Geometry check sheet. Reference: the model listing, model coordinates, mm. Give positions to 0.01 mm unless a question says otherwise; leave off trailing zeros. One line per item, written item: value. Start each with the question number.
(1) Sectioned sample at A-A, the plane z = 2.55. State how many separate pieces and enclosed holes the cut face has, then the cut area to 3 significant figures.
(2) Gauge pin test, flat ends, axial feed: pin 1 Ø1 at (y, z) = (102, 2.5) entering from +X; pin 2 Ø1.6 at (x, z) = (62, 1) entering from -Y; pin 3 Ø1 at (x, z) = (-61.5, 1) entering from +Y. Record the tip position at first contact, or that the pin passes through.
(3) Scan lines: line 1 along Y through (x, z) = (-54.5, 1.15); line 2 along X through (y, z) = (-150, 1.2). Record each from-to range of solid material in increasing order. Write a range as from..to.
from build123d import *

# Parameters (mm, degrees)
CROQUIS1_W              = 3.3
CROQUIS1_H              = 3.3
SALIENTE_EXTRUIR1_DEPTH = 3.3


with BuildPart() as part:
    # Croquis1 → Saliente-Extruir1 (new body)
    with BuildSketch(Plane.XY):
        Polygon((60, 27.9389154), (63.3, 27.9389154), (63.3, 19.9089154), (60, 19.9089154), (60, 11.03980694), (63.3, 11.03980694), (63.3, 3.00980694), (60, 3.00980694), (60, -3.00980694), (63.3, -3.00980694), (63.3, -11.03980694), (60, -11.03980694), (60, -19.9089154), (63.3, -19.9089154), (63.3, -27.9389154), (60, -27.9389154), (60, -36.80802386), (63.3, -36.80802386), (63.3, -44.83802386), (60, -44.83802386), (60, -53.70713232), (63.3, -53.70713232), (63.3, -61.73713232), (60, -61.73713232), (60, -70.60624078), (63.3, -70.60624078), (63.3, -78.63624078), (60, -78.63624078), (60, -87.50534924), (63.3, -87.50534924), (63.3, -95.53534924), (60, -95.53534924), (60, -104.4044577), (63.3, -104.4044577), (63.3, -112.4344577), (60, -112.4344577), (60, -121.30356616), (63.3, -121.30356616), (63.3, -129.33356616), (60, -129.33356616), (60, -138.20267462), (63.3, -138.20267462), (63.3, -146.23267462), (60, -146.23267462), (60, -155.10178308), (63.3, -155.10178308), (63.3, -163.13178308), (60, -163.13178308), (60, -172.00089154), (63.3, -172.00089154), (63.3, -180.03089154), (60, -180.03089154), (60, -188.9), (63.3, -188.9), (63.3, -196.93), (60, -196.93), (60, -200), (-60, -200), (-60, -196.93), (-63.3, -196.93), (-63.3, -188.9), (-60, -188.9), (-60, -180.03089154), (-63.3, -180.03089154), (-63.3, -172.00089154), (-60, -172.00089154), (-60, -163.13178308), (-63.3, -163.13178308), (-63.3, -155.10178308), (-60, -155.10178308), (-60, -146.23267462), (-63.3, -146.23267462), (-63.3, -138.20267462), (-60, -138.20267462), (-60, -129.33356616), (-63.3, -129.33356616), (-63.3, -121.30356616), (-60, -121.30356616), (-60, -112.4344577), (-63.3, -112.4344577), (-63.3, -104.4044577), (-60, -104.4044577), (-60, -95.53534924), (-63.3, -95.53534924), (-63.3, -87.50534924), (-60, -87.50534924), (-60, -78.63624078), (-63.3, -78.63624078), (-63.3, -70.60624078), (-60, -70.60624078), (-60, -61.73713232), (-63.3, -61.73713232), (-63.3, -53.70713232), (-60, -53.70713232), (-60, -44.83802386), (-63.3, -44.83802386), (-63.3, -36.80802386), (-60, -36.80802386), (-60, -27.9389154), (-63.3, -27.9389154), (-63.3, -19.9089154), (-60, -19.9089154), (-60, -11.03980694), (-63.3, -11.03980694), (-63.3, -3.00980694), (-60, -3.00980694), (-60, 3.00980694), (-63.3, 3.00980694), (-63.3, 11.03980694), (-60, 11.03980694), (-60, 19.9089154), (-63.3, 19.9089154), (-63.3, 27.9389154), (-60, 27.9389154), (-60, 36.80802386), (-63.3, 36.80802386), (-63.3, 44.83802386), (-60, 44.83802386), (-60, 53.70713232), (-63.3, 53.70713232), (-63.3, 61.73713232), (-60, 61.73713232), (-60, 70.60624078), (-63.3, 70.60624078), (-63.3, 78.63624078), (-60, 78.63624078), (-60, 87.50534924), (-63.3, 87.50534924), (-63.3, 95.53534924), (-60, 95.53534924), (-60, 104.4044577), (-63.3, 104.4044577), (-63.3, 112.4344577), (-60, 112.4344577), (-60, 121.30356616), (-63.3, 121.30356616), (-63.3, 129.33356616), (-60, 129.33356616), (-60, 138.20267462), (-63.3, 138.20267462), (-63.3, 146.23267462), (-60, 146.23267462), (-60, 155.10178308), (-63.3, 155.10178308), (-63.3, 163.13178308), (-60, 163.13178308), (-60, 172.00089154), (-63.3, 172.00089154), (-63.3, 180.03089154), (-60, 180.03089154), (-60, 188.9), (-63.3, 188.9), (-63.3, 196.93), (-60, 196.93), (-60, 200), (60, 200), (60, 196.93), (63.3, 196.93), (63.3, 188.9), (60, 188.9), (60, 180.03089154), (63.3, 180.03089154), (63.3, 172.00089154), (60, 172.00089154), (60, 163.13178308), (63.3, 163.13178308), (63.3, 155.10178308), (60, 155.10178308), (60, 146.23267462), (63.3, 146.23267462), (63.3, 138.20267462), (60, 138.20267462), (60, 129.33356616), (63.3, 129.33356616), (63.3, 121.30356616), (60, 121.30356616), (60, 112.4344577), (63.3, 112.4344577), (63.3, 104.4044577), (60, 104.4044577), (60, 95.53534924), (63.3, 95.53534924), (63.3, 87.50534924), (60, 87.50534924), (60, 78.63624078), (63.3, 78.63624078), (63.3, 70.60624078), (60, 70.60624078), (60, 61.73713232), (63.3, 61.73713232), (63.3, 53.70713232), (60, 53.70713232), (60, 44.83802386), (63.3, 44.83802386), (63.3, 36.80802386), (60, 36.80802386), align=None)
        with Locations((54.44567586, -101.72796576)):
            Rectangle(CROQUIS1_W, CROQUIS1_H, mode=Mode.SUBTRACT)
        with Locations((-54.44567586, -101.72796576)):
            Rectangle(CROQUIS1_W, CROQUIS1_H, mode=Mode.SUBTRACT)
        with Locations((-54.44567586, 101.72796576)):
            Rectangle(CROQUIS1_W, CROQUIS1_H, mode=Mode.SUBTRACT)
        with Locations((54.44567586, 101.72796576)):
            Rectangle(CROQUIS1_W, CROQUIS1_H, mode=Mode.SUBTRACT)
    extrude(amount=SALIENTE_EXTRUIR1_DEPTH)


solid = part.part
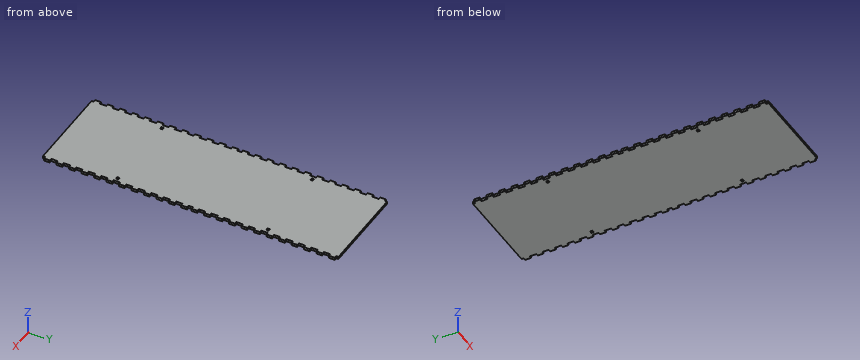
Calculated:
1. separate pieces: 1
1. enclosed holes: 4
1. area: 49,200 mm2
2. pin 1: stops at x = 60
2. pin 2: stops at y = -196.93
2. pin 3: stops at y = 196.93
3. line 1: y = -200..-103.38, -100.08..100.08, 103.38..200
3. line 2: x = -60..60
